The model under review builds one solid part; all positions refer to its coordinate system, in mm. A direction names the side the tool comes from. Round coordinates to 2 decimals unless told otherwise and drop trailing zeros. Write each loop counter-clockwise with the first axis right and the second up, starting at its lowest first coordinate (ties: lowest second). Pieces come first, ordered by that corner, then holes. Notation, with made-up numbers: (-30.5, 12) - (-21.5, 12) arc R25 cw to (-21.5, 44) - close; hole circle Ø3 at (71, 32). An arc over 180 degrees is marked (long way). Write each question's results on one line, items separated by ' | '.
```python
from build123d import *

# Parameters (mm, degrees)
BOSS_EXTRUDE2_DEPTH = 13
FILLET1_R           = 2.5
CUT_EXTRUDE1_DEPTH  = 13
SKETCH4_R           = 1.5
SKETCH4_R_2         = 3.9
CUT_EXTRUDE2_DEPTH  = 13
SKETCH5_R           = 1.5
SKETCH5_R_2         = 5
CUT_EXTRUDE3_DEPTH  = 13


with BuildPart() as part:
    # Sketch1 → Boss-Extrude2 (new, symmetric)
    with BuildSketch(Plane.XY):
        with BuildLine():
            Line((0, 2.5), (0, 33))
            Line((0, 33), (3, 33))
            Line((3, 33), (3, 5.5))
            ThreePointArc((3, 5.5), (3.732233047, 3.732233047), (5.5, 3))
            Line((5.5, 3), (31, 3))
            Line((31, 3), (31, 0))
            Line((31, 0), (2.5, 0))
            ThreePointArc((2.5, 0), (0.732233047, 0.732233047), (0, 2.5))
        make_face()
    extrude(amount=BOSS_EXTRUDE2_DEPTH, both=True)

    # Fillet1
    fillet1_edges = [part.edges().sort_by_distance(p)[0] for p in [
        (31, 1.5, 13),
        (31, 1.5, -13),
    ]]
    fillet(fillet1_edges, radius=FILLET1_R)

    # Sketch3 → Cut-Extrude1 (cut, symmetric)
    with BuildSketch(Plane(origin=(3, 0, 0), x_dir=(0, 0, -1), z_dir=(1, 0, 0))):
        with BuildLine():
            Line((-13, 33), (-13, 20))
            ThreePointArc((-13, 20), (-9.192388155, 29.192388155), (0, 33))
            Line((0, 33), (-13, 33))
        make_face()
        with BuildLine():
            Line((13, 33), (0, 33))
            ThreePointArc((0, 33), (9.192388155, 29.192388155), (13, 20))
            Line((13, 20), (13, 33))
        make_face()
    extrude(amount=CUT_EXTRUDE1_DEPTH, both=True, mode=Mode.SUBTRACT)

    # Sketch4 → Cut-Extrude2 (cut, symmetric)
    with BuildSketch(Plane(origin=(3, 0, 0), x_dir=(0, 0, -1), z_dir=(1, 0, 0))):
        with Locations(Location((-8.5, 20, 0), (0, 0, 90))):
            Circle(SKETCH4_R)
        with Locations(Location((8.5, 20, 0), (0, 0, 90))):
            Circle(SKETCH4_R)
        with Locations(Location((0, 20, 0), (0, 0, 90))):
            Circle(SKETCH4_R_2)
    extrude(amount=CUT_EXTRUDE2_DEPTH, both=True, mode=Mode.SUBTRACT)

    # Sketch5 → Cut-Extrude3 (cut, symmetric)
    with BuildSketch(Plane.XZ):
        with Locations(Location((23.75, 8, 0), (0, 0, 270))):
            Circle(SKETCH5_R)
        with Locations(Location((23.75, -8, 0), (0, 0, 270))):
            Circle(SKETCH5_R)
        with Locations(Location((9.75, 8, 0), (0, 0, 270))):
            Circle(SKETCH5_R)
        with Locations(Location((9.75, -8, 0), (0, 0, 270))):
            Circle(SKETCH5_R)
        with Locations(Location((16.780453702, 0, 0), (0, 0, 270))):
            Circle(SKETCH5_R_2)
    extrude(amount=CUT_EXTRUDE3_DEPTH, both=True, mode=Mode.SUBTRACT)


solid = part.part
```
Q1. We need section A-A (x = 23.75). State the section outline as (y, z) points.
Evaluation:
outline: (0, -13) - (3, -13) - (3, -9.5) - (0, -9.5) - close; (0, -6.5) - (3, -6.5) - (3, 6.5) - (0, 6.5) - close; (0, 9.5) - (3, 9.5) - (3, 13) - (0, 13) - close
Q2. We need section C-C (z = 8.5). State the section outline as (x, y) points, plus the area to 3 significant figures.
Evaluation:
outline: (0, 2.5) arc R2.5 ccw to (2.5, 0) - (8.34, 0) - (8.34, 3) - (5.5, 3) arc R2.5 cw to (3, 5.5) - (3, 18.5) - (0, 18.5) - close; (0, 21.5) - (3, 21.5) - (3, 29.84) - (0, 29.84) - close; (11.16, 0) - (22.34, 0) - (22.34, 3) - (11.16, 3) - close; (25.16, 0) - (31, 0) - (31, 3) - (25.16, 3) - close | area: 148 mm^2
Q3. Insertion check: P1, Ø12, axis at x = 26, z = 10, coming from the -Y side; P2, Ø2.5, axis at x = 23.75, z = -8, coming from the +Y side; P3, Ø4, axis at y = 20, z = -8.5, coming from the +X side; P4, Ø7.5, axis at x = 23, z = -1, coming from the +Y side. Each pin has a flat end and moves straight along its axis. Give the tip position at first contact, or say it passes through.
Evaluation:
P1: stops at y = 0 | P2: passes through | P3: stops at x = 3 | P4: stops at y = 3
Q4. The part is to be moulded in two halves that separate along X. For faces 1 (the flat face through (0, 14, 0)), 2 (the cylindrical face through (1.52, 18.5, -8.43)), 3 (the cylindrical face through (25.237, 1.479, 8.195)), 4 (the cylindrical face through (21.74, 1.48, 0.65)), say which applies: released by +X, released by -X, zero draft, split by the parting line, or undercut.
Evaluation:
face 1: released by -X | face 2: zero draft | face 3: undercut | face 4: undercut
Q5. For probe 1 along Z at (x, y) = (2.4, 20); probe 2 along X at (y, z) = (2.35, 8); probe 3 along Z at (x, y) = (23, 1), list the stretches that pass through material, from the lowest coordinate up.
Evaluation:
probe 1: z = -13 to -10, -7 to -3.9, 3.9 to 7, 10 to 13 | probe 2: x = 0 to 8.25, 11.25 to 22.25, 25.25 to 31 | probe 3: z = -13 to -9.3, -6.7 to 6.7, 9.3 to 13
Q6. We need section D-D (x = 27). State the section outline as (y, z) points, plus the area to 3 significant figures.
Evaluation:
outline: (0, -13) - (3, -13) - (3, 13) - (0, 13) - close | area: 78.0 mm^2
Q7. We need section B-B (z = 2). State the section outline as (x, y) points.
Evaluation:
outline: (0, 2.5) arc R2.5 ccw to (2.5, 0) - (12.2, 0) - (12.2, 3) - (5.5, 3) arc R2.5 cw to (3, 5.5) - (3, 16.65) - (0, 16.65) - close; (0, 23.35) - (3, 23.35) - (3, 32.85) - (0, 32.85) - close; (21.36, 0) - (31, 0) - (31, 3) - (21.36, 3) - close
Q8. Tool access review of faces 5 (the cylindrical face through (0.752, 0.713, 0.182)), 6 (the flat face through (3, 16, -3)): name each direction out of +Z, -Z, +X, -X, +Y, -Y from which nothing blocks a thin tool from reaching the whole face with its end or side.
Evaluation:
face 5: +Z, -Z, -X, -Y | face 6: +Z, -Z, +X, +Y
